Could you check a few things on this model? Use its own coordinates, in mm. Face numbers are marked on the shaded views. A direction names the side the tool comes from. Give positions to 0.01 mm unless a question says otherwise; leave off trailing zeros. Order: outer loops, then holes, each group sorted by start corner. A loop starts at its lowest first (then second) coordinate and runs counter-clockwise, first axis right, second up.
(1) On a 3-axis mill with a long thin cutter (end or side, diameter ignored), from which of +Z, -Z, +X, -X, +Y, -Y can I reach the whole of each face in a straight line? I mean the marked faces 1, 2 and 3. Say none if no direction works.
(2) Will these pins go through, and if not, where does the flat tip stop? pin 1 (8 mm diameter, centred on x = 65.5, y = 11.5, fed in from -Z); pin 2 (1.5 mm diameter, centred on x = 44.5, y = 4.5, fed in from +Z); pin 3 (2 mm diameter, centred on x = 93.5, y = 7, fed in from -Z).
(3) Imagine slicing it at C-C, the plane y = 33. Write out the boundary of the cut face in (x, z).
(4) If we mould it in two halves opening along X, with no side actions, what happens to the marked faces 4, 5 and 6? For each: released by +X, released by -X, zero draft, split by the parting line, or undercut.
(5) Imagine slicing it at A-A, the plane x = 73.25. Write out the boundary of the cut face in (y, z).
(6) Imagine slicing it at D-D, the plane y = 10. Write out the boundary of the cut face in (x, z), then the cut area to 3 significant figures.
(7) If I drill on probe 1 along X at (y, z) = (15, -25); probe 2 along Z at (x, y) = (72, 19); probe 3 along Z at (x, y) = (73.25, 16), over which ranges is the centre line in solid material (lowest first)?
(8) Imagine slicing it at B-B, the plane z = -25. Write out the boundary of the cut face in (x, y).
from build123d import *

# Parameters (mm, degrees)
SKETCH1_R               = 3
BOSS_EXTRUDE2_DEPTH     = 35
CUT_EXTRUDE1_DEPTH      = 128.625428501
CUT_EXTRUDE1_DEPTH_BACK = 128.625428501


with BuildPart() as part:
    # Sketch1 → Boss-Extrude2 (new body)
    with BuildSketch(Plane(origin=(0, 0, 0), x_dir=(1, 0, 0), z_dir=(0, 1, 0))):
        Polygon((0, 0), (25.3, 0), (25.3, -2), (28.8, -2), (28.8, 0), (77.7, 0), (77.7, -2), (81.2, -2), (81.2, 0), (106.5, 0), (106.5, 61), (0, 61), align=None)
        with Locations(Location((33.25, 25, 0), (0, 0, 270))):
            Circle(SKETCH1_R, mode=Mode.SUBTRACT)
        with Locations(Location((73.25, 25, 0), (0, 0, 90))):
            Circle(SKETCH1_R, mode=Mode.SUBTRACT)
    extrude(amount=BOSS_EXTRUDE2_DEPTH)

    # Sketch2 → Cut-Extrude1 (cut, two sides: drawn at the far end of the back side and taken through both)
    with BuildSketch(Plane.ZY.offset(-CUT_EXTRUDE1_DEPTH_BACK)):
        Polygon((-61, 35), (-58, 35), (-61, 0), align=None)
    extrude(amount=CUT_EXTRUDE1_DEPTH + CUT_EXTRUDE1_DEPTH_BACK, mode=Mode.SUBTRACT)


solid = part.part
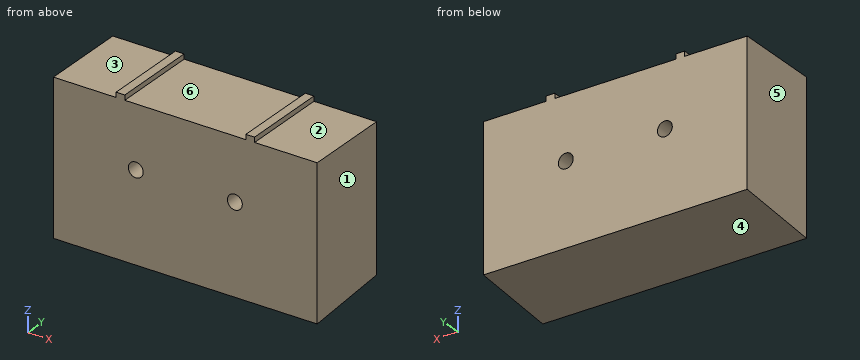
Answer block:
1. face 1: +Z, -Z, +X, +Y, -Y
1. face 2: +Z, +X, +Y, -Y
1. face 3: +Z, -X, +Y, -Y
2. pin 1: stops at z = -60.36
2. pin 2: stops at z = 0
2. pin 3: stops at z = -60.49
3. outline: (0, -58.17) - (106.5, -58.17) - (106.5, 0) - (81.2, 0) - (81.2, 2) - (77.7, 2) - (77.7, 0) - (28.8, 0) - (28.8, 2) - (25.3, 2) - (25.3, 0) - (0, 0) - close; hole circle Ø6 at (33.25, -25); hole circle Ø6 at (73.25, -25)
4. face 4: zero draft
4. face 5: released by -X
4. face 6: undercut
5. outline: (0, -61) - (35, -58) - (35, -28) - (0, -28) - close; (0, -22) - (35, -22) - (35, 0) - (0, 0) - close
6. outline: (0, -60.14) - (106.5, -60.14) - (106.5, 0) - (81.2, 0) - (81.2, 2) - (77.7, 2) - (77.7, 0) - (28.8, 0) - (28.8, 2) - (25.3, 2) - (25.3, 0) - (0, 0) - close; hole circle Ø6 at (33.25, -25); hole circle Ø6 at (73.25, -25)
6. area: 6,360 mm2
7. probe 1: x = 0 to 30.25, 36.25 to 70.25, 76.25 to 106.5
7. probe 2: z = -59.37 to -27.73, -22.27 to 0
7. probe 3: z = -59.63 to -28, -22 to 0
8. outline: (0, 0) - (30.25, 0) - (30.25, 35) - (0, 35) - close; (36.25, 0) - (70.25, 0) - (70.25, 35) - (36.25, 35) - close; (76.25, 0) - (106.5, 0) - (106.5, 35) - (76.25, 35) - close
